Build history of the part. All positions in model axes, mm. Face numbers are marked on the shaded views. A direction names the side the tool comes from. Give positions to 0.01 mm unless a question says otherwise; leave off trailing zeros. Order: outer loops, then holes, each group sorted by start corner. A loop starts at its lowest first (then second) coordinate and runs counter-clockwise, first axis right, second up. Notation, with made-up numbers: (43.5, 68.5) -> (75.5, 68.5) arc R30 ccw to (75.5, 105.5) -> close; hole circle Ø10 at (43.5, -27). An arc over 180 degrees is marked (long way). Write item = value, one per line. Start each with the question number.
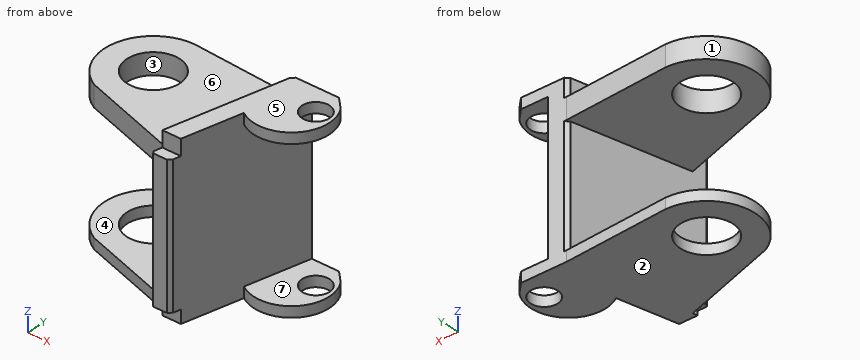
from build123d import *
from OCP.BRepFilletAPI import BRepFilletAPI_MakeChamfer

# Parameters (mm, degrees)
BOSS_EXTRU_1_DEPTH      = 320
ENL_V_MAT_EXTRU_1_DEPTH = 30
ENL_V_START             = -295
ENL_V_MAT_EXTRU_2_DEPTH = 25
ESQUISSE5_R             = 26
BOSS_EXTRU_2_DEPTH      = 20
BOSS_EXTRU_3_START      = -35
ESQUISSE5_3_R           = 50
BOSS_EXTRU_3_DEPTH      = 40
BOSS_EXTRU_4_START      = -300
ESQUISSE5_5_R           = 50
BOSS_EXTRU_4_DEPTH      = 20
BOSS_EXTRU_5_START      = -300
ESQUISSE5_6_R           = 26
BOSS_EXTRU_5_DEPTH      = 20
CHANFREIN1_SIZE         = 5
CHANFREIN1_SIZE_2       = 6.671835022
CHANFREIN2_SIZE         = 5
CHANFREIN2_SIZE2        = 6.671835022
CHANFREIN2_SIZE2_2      = 4.169025226
CHANFREIN5_START        = 181.632019665
CHANFREIN5_OUTLINE_W    = 32
CHANFREIN5_OUTLINE_H    = 22
CHANFREIN5_DEPTH        = 2.367980335
CHANFREIN6_START        = 181.632019665
CHANFREIN6_OUTLINE_W    = 32
CHANFREIN6_OUTLINE_H    = 22
CHANFREIN6_DEPTH        = 2.367980335


with BuildPart() as part:
    # Esquisse1 → Boss.-Extru.1 (new body)
    with BuildSketch(Plane.XY):
        Polygon((10.109909982, 160.217391304), (45.109909982, 160.217391304), (-12.607137799, -89.782608696), (-47.607137799, -89.782608696), align=None)
    extrude(amount=BOSS_EXTRU_1_DEPTH)

    # Esquisse2 → Enlèv. mat.-Extru.1 (cut)
    with BuildSketch(Plane.XY.offset(320)):
        Polygon((-47.607137799, -89.782608696), (-42.989773977, -69.782608696), (-7.989773977, -69.782608696), (-12.607137799, -89.782608696), align=None)
    extrude(amount=-ENL_V_MAT_EXTRU_1_DEPTH, mode=Mode.SUBTRACT)

    # Esquisse3 → Enlèv. mat.-Extru.2 (cut)
    with BuildSketch(Plane.XY.offset(320).offset(ENL_V_START)):
        Polygon((-47.607137799, -89.782608696), (-42.989773977, -69.782608696), (-7.989773977, -69.782608696), (-12.607137799, -89.782608696), align=None)
    extrude(amount=-ENL_V_MAT_EXTRU_2_DEPTH, mode=Mode.SUBTRACT)

    # Esquisse5 → Boss.-Extru.2 (add)
    with BuildSketch(Plane.XY.offset(320)):
        with BuildLine():
            Line((96.899074267, 160.217391304), (45.109909982, 160.217391304))
            Line((45.109909982, 160.217391304), (17.591978342, 41.024134293))
            ThreePointArc((17.591978342, 41.024134293), (116.84215481, 60.967214836), (96.899074267, 160.217391304))
        make_face()
        with Locations((95.109909982, 110.217391304)):
            Circle(ESQUISSE5_R, mode=Mode.SUBTRACT)
    extrude(amount=-BOSS_EXTRU_2_DEPTH)

    # Esquisse5<3> → Boss.-Extru.3 (add)
    with BuildSketch(Plane.XY.offset(320).offset(BOSS_EXTRU_3_START)):
        with BuildLine():
            Line((-230.213971145, -0.950262244), (-40.985726083, -61.102123595))
            Line((-40.985726083, -61.102123595), (10.109909982, 160.217391304))
            Line((10.109909982, 160.217391304), (-187.731895981, 173.717391304))
            ThreePointArc((-187.731895981, 173.717391304), (-277.611698921, 103.077652588), (-230.213971145, -0.950262244))
        make_face()
        with Locations((-187.731895981, 81.217391304)):
            Circle(ESQUISSE5_3_R, mode=Mode.SUBTRACT)
    extrude(amount=-BOSS_EXTRU_3_DEPTH)

    # Esquisse5<5> → Boss.-Extru.4 (add)
    with BuildSketch(Plane.XY.offset(320).offset(BOSS_EXTRU_4_START)):
        with BuildLine():
            Line((-230.213971145, -0.950262244), (-40.985726083, -61.102123595))
            Line((-40.985726083, -61.102123595), (10.109909982, 160.217391304))
            Line((10.109909982, 160.217391304), (-187.731895981, 173.717391304))
            ThreePointArc((-187.731895981, 173.717391304), (-277.611698921, 103.077652588), (-230.213971145, -0.950262244))
        make_face()
        with Locations((-187.731895981, 81.217391304)):
            Circle(ESQUISSE5_5_R, mode=Mode.SUBTRACT)
    extrude(amount=-BOSS_EXTRU_4_DEPTH)

    # Esquisse5<6> → Boss.-Extru.5 (add)
    with BuildSketch(Plane.XY.offset(320).offset(BOSS_EXTRU_5_START)):
        with BuildLine():
            Line((96.899074267, 160.217391304), (45.109909982, 160.217391304))
            Line((45.109909982, 160.217391304), (17.591978342, 41.024134293))
            ThreePointArc((17.591978342, 41.024134293), (116.84215481, 60.967214836), (96.899074267, 160.217391304))
        make_face()
        with Locations((95.109909982, 110.217391304)):
            Circle(ESQUISSE5_6_R, mode=Mode.SUBTRACT)
    extrude(amount=-BOSS_EXTRU_5_DEPTH)

    # Chanfrein1
    # the kernel refuses this chamfer: 6.671835022, 5 mm, written as the material it takes off along each edge
    with BuildSketch(Plane(origin=(10.109909982, 160.217391304, 20), x_dir=(1, 0, 0), z_dir=(0, 0, 1))) as chanfrein1_piece_1:
        Polygon((CHANFREIN1_SIZE, 0), (-CHANFREIN1_SIZE_2 * 0.224951054343, -CHANFREIN1_SIZE_2 * 0.974370064782), (0, 0), align=None)
    extrude(amount=225, mode=Mode.SUBTRACT)
    with BuildSketch(Plane(origin=(10.109909982, 160.217391304, 285), x_dir=(1, 0, 0), z_dir=(0, 0, 1))) as chanfrein1_piece_2:
        Polygon((CHANFREIN1_SIZE, 0), (-CHANFREIN1_SIZE_2 * 0.224951054343, -CHANFREIN1_SIZE_2 * 0.974370064782), (0, 0), align=None)
    extrude(amount=52.24901503, mode=Mode.SUBTRACT)

    # Chanfrein2: one chamfer whose edges measure the first distance from different faces: ONE call of the kernel's chamfer builder (chamfer() names one face for all edges)
    chanfrein2_edges_1 = [part.edges().sort_by_distance(p)[0] for p in [
        (-12.607137799, -89.782608696, 157.5),
    ]]
    chanfrein2_side_1 = [part.faces().sort_by_distance(p)[0] for p in [
        (-30.107137799, -89.782608696, 157.5),
    ]]
    chanfrein2_edges_2 = [part.edges().sort_by_distance(p)[0] for p in [
        (-47.607137799, -89.782608696, 157.5),
    ]]
    chanfrein2_side_2 = [part.faces().sort_by_distance(p)[0] for p in [
        (-19.722598228, 30.998601722, 155.760522115),
    ]]
    chanfrein2 = BRepFilletAPI_MakeChamfer(part.part.solid().wrapped)
    for e in chanfrein2_edges_1:
        chanfrein2.Add(CHANFREIN2_SIZE, CHANFREIN2_SIZE2, e.wrapped, chanfrein2_side_1[0].wrapped)  # the first distance lies on this face
    for e in chanfrein2_edges_2:
        chanfrein2.Add(CHANFREIN2_SIZE, CHANFREIN2_SIZE2_2, e.wrapped, chanfrein2_side_2[0].wrapped)  # the first distance lies on this face
    add(Compound.cast(chanfrein2.Shape()), mode=Mode.REPLACE)

    # Chanfrein5: read off the stored shape, not the designer's step
    # Chanfrein5 outline → Chanfrein5 (cut)
    with BuildSketch(Plane(origin=(0, 0, 0), x_dir=(0.7071067811865471, -0.707106781186548, 0), z_dir=(0.707106781186548, 0.707106781186547, 0)).offset(CHANFREIN5_START)):
        with Locations((-30, -310)):
            Rectangle(CHANFREIN5_OUTLINE_W, CHANFREIN5_OUTLINE_H)
    extrude(amount=CHANFREIN5_DEPTH, mode=Mode.SUBTRACT)

    # Chanfrein6: read off the stored shape, not the designer's step
    # Chanfrein6 outline → Chanfrein6 (cut)
    with BuildSketch(Plane(origin=(0, 0, 0), x_dir=(0.707106781186546, -0.707106781186549, 0), z_dir=(0.707106781186549, 0.707106781186546, 0)).offset(CHANFREIN6_START)):
        with Locations((-30, -10)):
            Rectangle(CHANFREIN6_OUTLINE_W, CHANFREIN6_OUTLINE_H)
    extrude(amount=CHANFREIN6_DEPTH, mode=Mode.SUBTRACT)


solid = part.part
(1) Wall check: line 1 (Z direction, x = -26.5, y = 87); line 2 (X direction, y = 100.5, z = 14); line 3 (Y direction, x = -190, z = 268.5). Give the ranges that are in metal, low to high. Write a range as [from, to].
(2) Cut at D-D, the plane x = -155.5. Give the cut face in (y, z), plus the area to 3 significant figures.
(3) Cut at B-B, the plane y = 124. Give the number of separate pieces and of enclosed holes in the cut face, plus the area to 3 significant figures.
(4) Cut at C-C, the plane z = 106. Give the cut face in (x, y), plus the area to 3 significant figures.
(5) 3-axis set-ups, long thin cutter, end or side, ignore diameter. For the marked faces 4, 5, 6 and 7: which of +Z, -Z, +X, -X, +Y, -Y reach the whole face in a straight line?
(6) Flat gauge pins, fed straight in: P1, Ø1.5, axis at y = -21.5, z = 158, coming from the +X side; P2, Ø16, axis at x = -20.5, y = -77, coming from the +Z side; P3, Ø3, axis at x = -79, z = 251.5, coming from the -Y side; P4, Ø12.5, axis at x = -20, z = 13, coming from the -Y side. Where does each tip first touch, or does it go through?
(7) Mould opens along Y. For the marked faces 1, 2 and 3 say: released by +Y, released by -Y, zero draft, split by the parting line, or undercut.
(8) Cut at A-A, the plane x = -95. Give the cut face in (y, z).
Results:
q1.line_1 = [0, 20], [245, 285]
q1.line_2 = [-278.2, -233.86], [-141.6, 70.99], [119.23, 128.83]
q1.line_3 = [-13.73, 31.27], [131.17, 173.69]
q2.outline = (-24.7, 0) -> (42.99, 0) -> (42.99, 20) -> (-24.7, 20) -> close; (-24.7, 245) -> (42.99, 245) -> (42.99, 285) -> (-24.7, 285) -> close; (119.44, 0) -> (171.52, 0) -> (171.52, 20) -> (119.44, 20) -> close; (119.44, 245) -> (171.52, 245) -> (171.52, 285) -> (119.44, 285) -> close
q2.area = 7,190 mm2
q3.separate_pieces = 5
q3.enclosed_holes = 0
q3.area = 26,100 mm2
q4.outline = (-46.48, -84.91) -> (-43.44, -89.78) -> (-17.61, -89.78) -> (-11.11, -83.28) -> (45.11, 160.22) -> (15.11, 160.22) -> (8.61, 153.72) -> close
q4.area = 8,710 mm2
q5.face_4 = -X, +Y
q5.face_5 = +Z, +X, -X, +Y, -Y
q5.face_6 = +Z, -X, +Y
q5.face_7 = +X, -Y
q6.P1 = 3.33
q6.P2 = 320
q6.P3 = -49.49
q6.P4 = -69.78
q7.face_1 = split by the parting line
q7.face_2 = zero draft
q7.face_3 = undercut
q8.outline = (-43.93, 0) -> (167.39, 0) -> (167.39, 20) -> (-43.93, 20) -> close; (-43.93, 245) -> (167.39, 245) -> (167.39, 285) -> (-43.93, 285) -> close
